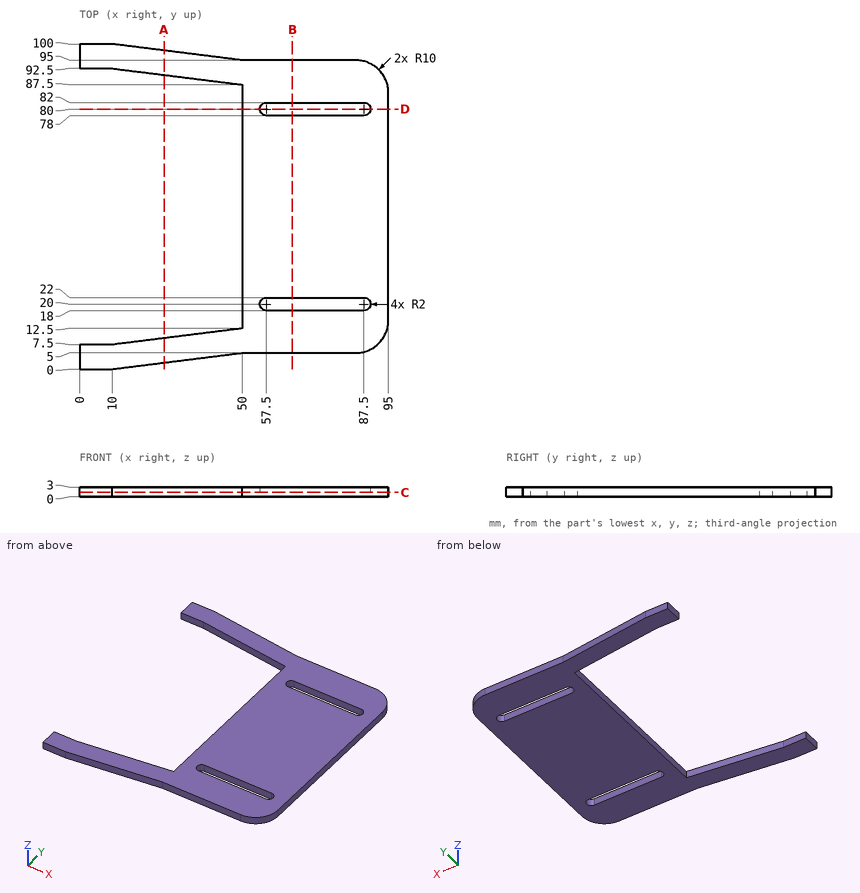
Verification items for this drawing (mm, ordinates from the low corner). Give positions to 0.01 mm unless a question says otherwise; leave off trailing zeros. Write each loop counter-clockwise with the first axis right and the second up, starting at its lowest first coordinate (ties: lowest second). Pieces come first, ordered by that corner, then holes.
1) Section check D-D, the plane y = 80. Record the boundary of the cut face in (x, z), and give its area (3 significant figures).
2) Gauge pin test, flat ends, axial feed: pin 1 (0.9 mm diameter, centred on x = 66, z = 2, fed in from -Y); pin 2 (1.5 mm diameter, centred on x = 79, z = 1.5, fed in from +Y); pin 3 (0.9 mm diameter, centred on y = 54.5, z = 1.5, fed in from -X). Record the tip position at first contact, or that the pin passes through.
3) Material ranges on L1, parallel to Y at x = 71.5, z = 1.8; L2, parallel to X at y = 72.5, z = 2.4; L3, parallel to Y at x = 30, z = 1.9, recorded low to high.
4) Section check B-B, the plane x = 65.5. Record the boundary of the cut face in (y, z).
5) Section check C-C, the plane z = 1.35. Record the boundary of the cut face in (x, y).
6) Section check A-A, the plane x = 26. Record the boundary of the cut face in (y, z), and give its area (3 significant figures).
Computed:
1. outline: (50, 0) - (55.5, 0) - (55.5, 3) - (50, 3) - close; (89.5, 0) - (95, 0) - (95, 3) - (89.5, 3) - close
1. area: 33.0 mm2
2. pin 1: stops at y = 5
2. pin 2: stops at y = 95
2. pin 3: stops at x = 50
3. L1: y = 5 to 18, 22 to 78, 82 to 95
3. L2: x = 50 to 95
3. L3: y = 2.5 to 10, 90 to 97.5
4. outline: (5, 0) - (18, 0) - (18, 3) - (5, 3) - close; (22, 0) - (78, 0) - (78, 3) - (22, 3) - close; (82, 0) - (95, 0) - (95, 3) - (82, 3) - close
5. outline: (0, 0) - (10, 0) - (50, 5) - (85, 5) arc R10 ccw to (95, 15) - (95, 85) arc R10 ccw to (85, 95) - (50, 95) - (10, 100) - (0, 100) - (0, 92.5) - (10, 92.5) - (50, 87.5) - (50, 12.5) - (10, 7.5) - (0, 7.5) - close; hole (57.5, 18) - (87.5, 18) arc R2 ccw to (87.5, 22) - (57.5, 22) arc R2 ccw to start; hole (57.5, 78) - (87.5, 78) arc R2 ccw to (87.5, 82) - (57.5, 82) arc R2 ccw to start
6. outline: (2, 0) - (9.5, 0) - (9.5, 3) - (2, 3) - close; (90.5, 0) - (98, 0) - (98, 3) - (90.5, 3) - close
6. area: 45.0 mm2
